```python
from build123d import *

# Parameters (mm, degrees)
SKETCH1_R           = 12.11
BOSS_EXTRUDE1_DEPTH = 31
FILLET1_R           = 1
SKETCH2_R           = 11.71
CUT_EXTRUDE1_DEPTH  = 1
SKETCH3_R           = 12.475
BOSS_EXTRUDE2_DEPTH = 4.36
SKETCH4_R           = 12.375
BOSS_EXTRUDE3_DEPTH = 8.3
SKETCH5_R           = 12.475
BOSS_EXTRUDE4_DEPTH = 4.43
SKETCH6_R           = 1.4
CUT_EXTRUDE2_DEPTH  = 6


with BuildPart() as part:
    # Sketch1 → Boss-Extrude1 (new body)
    with BuildSketch(Plane(origin=(0, 0, 0), x_dir=(0, 0, -1), z_dir=(1, 0, 0))):
        Circle(SKETCH1_R)
    extrude(amount=BOSS_EXTRUDE1_DEPTH)

    # Fillet1
    fillet1_edges = [part.edges().sort_by_distance(p)[0] for p in [
        (0, 0, 12.11),
    ]]
    fillet(fillet1_edges, radius=FILLET1_R)

    # Sketch2 → Cut-Extrude1 (cut)
    with BuildSketch(Plane(origin=(31, 0, 0), x_dir=(0, 0, -1), z_dir=(1, 0, 0))):
        Circle(SKETCH2_R)
    extrude(amount=-CUT_EXTRUDE1_DEPTH, mode=Mode.SUBTRACT)

    # Sketch3 → Boss-Extrude2 (add)
    with BuildSketch(Plane.ZY):
        Circle(SKETCH3_R)
    extrude(amount=BOSS_EXTRUDE2_DEPTH)

    # Sketch4 → Boss-Extrude3 (add)
    with BuildSketch(Plane.ZY.offset(4.36)):
        Circle(SKETCH4_R)
    extrude(amount=BOSS_EXTRUDE3_DEPTH)

    # Sketch5 → Boss-Extrude4 (add)
    with BuildSketch(Plane.ZY.offset(12.66)):
        Circle(SKETCH5_R)
    extrude(amount=BOSS_EXTRUDE4_DEPTH)

    # Sketch6 → Cut-Extrude2 (cut)
    with BuildSketch(Plane.ZY.offset(17.09)):
        with Locations((0, 8.5)):
            Circle(SKETCH6_R)
        with Locations((0, -8.5)):
            Circle(SKETCH6_R)
    extrude(amount=-CUT_EXTRUDE2_DEPTH, mode=Mode.SUBTRACT)


solid = part.part
```
The model under review builds one solid part; all positions refer to its coordinate system, in mm. A direction names the side the tool comes from. Round coordinates to 2 decimals unless told otherwise and drop trailing zeros. Loops run counter-clockwise (first coordinate to the right, second up) from the corner with the lowest first, then second, coordinate; pieces in that order, holes last. Notation, with made-up numbers: (-24.75, 28) -> (0.25, 28) arc R7 cw to (0.25, 38) -> close; hole circle Ø1 at (2, -33.5). An arc over 180 degrees is marked (long way). Answer as a JSON object with one key per item and string values. Group by question number.
1) We need section C-C on x = -2.5. Write out the cut boundary in (y, z) (3 decimals), then the cut area to 3 significant figures.
2) For pin 1 Ø12.5 at (y, z) = (5.5, 3) entering from +X; pin 2 Ø5 at (x, y) = (24, -2.5) entering from -Z; pin 3 Ø0.8 at (y, z) = (-8.5, 0) entering from -X; pin 4 Ø4 at (x, z) = (18, 8.5) entering from +Y, all flat-tipped, find the tip position at first contact; note any pin that passes through.
3) We need section A-A on y = 0. Write out the cut boundary in (x, z) (3 decimals).
4) For faces 5 (the face through (-14.132, 7.133, -0.303)), 6 (the face through (15.79, -7.37, 9.61)), 7 (the face through (-17.09, 0, 0)), list the 3-axis set-ups (+Z, -Z, +X, -X, +Y, -Y) from which the entire face can be reached by the end or side of a thin tool; tool diameter is ignored.
5) Mouldability with a two-part tool opening along X and no side actions: class faces 1 (the face through (-8.45, 12.27, -1.61)), 2 (the face through (30, 0, 0)), 3 (the face through (-11.09, -8, 0)), 4 (the face through (-14.132, -9.867, -0.303)) as released by +X, released by -X, zero draft, split by the parting line, or undercut.
6) We need section D-D on x = 8. Write out the cut boundary in (y, z), then the cut area to 3 significant figures.
7) For line 1 (Y direction, x = -12.35, z = 0) (3 decimals); line 2 (Y direction, x = -14.25, z = 0) (3 decimals); line 3 (Y direction, x = 30.35, z = 0), list the stretches that pass through material, from the lowest coordinate up. Write a range as [from, to].
Result set:
{
 "1": {"outline": "circle Ø24.95 at (0, 0)", "area": "489 mm²"},
 "2": {"pin 1": "x = 31", "pin 2": "z = -12.11", "pin 3": "x = -11.09", "pin 4": "y = 10.22"},
 "3": {"outline": "(-17.09, -12.475) -> (-12.66, -12.475) -> (-12.66, -12.375) -> (-4.36, -12.375) -> (-4.36, -12.475) -> (0, -12.475) -> (0, -11.11) arc R1 ccw to (1, -12.11) -> (31, -12.11) -> (31, -11.71) -> (30, -11.71) -> (30, 11.71) -> (31, 11.71) -> (31, 12.11) -> (1, 12.11) arc R1 ccw to (0, 11.11) -> (0, 12.475) -> (-4.36, 12.475) -> (-4.36, 12.375) -> (-12.66, 12.375) -> (-12.66, 12.475) -> (-17.09, 12.475) -> close"},
 "4": {"face 5": "-X", "face 6": "+X", "face 7": "+Z, -Z, -X, +Y, -Y"},
 "5": {"face 1": "undercut", "face 2": "released by +X", "face 3": "released by -X", "face 4": "zero draft"},
 "6": {"outline": "circle Ø24.22 at (0, 0)", "area": "461 mm²"},
 "7": {"line 1": "[-12.375, -9.9], [-7.1, 7.1], [9.9, 12.375]", "line 2": "[-12.475, -9.9], [-7.1, 7.1], [9.9, 12.475]", "line 3": "[-12.11, -11.71], [11.71, 12.11]"}
}
